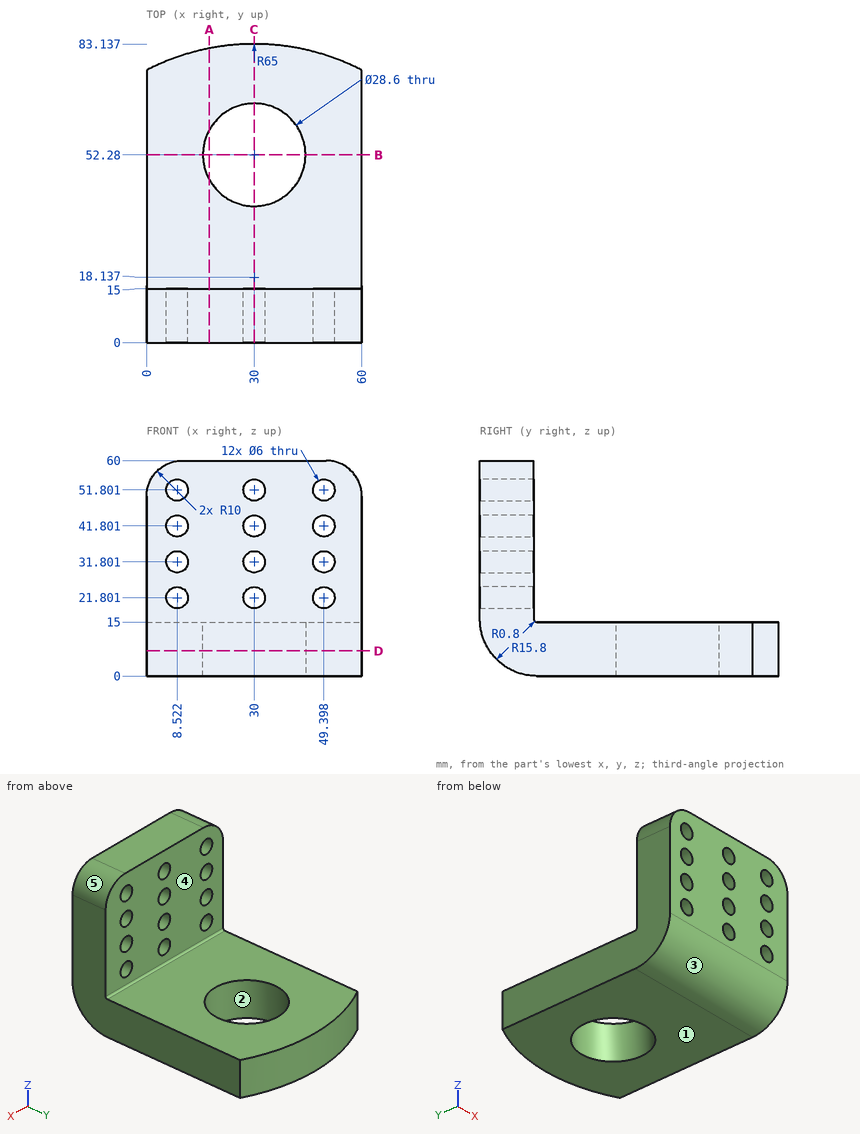
Source: three-view drawing plus pictorial views. Frame: mm from the lowest corner of the part. A direction names the side the tool comes from. Round coordinates to 2 decimals unless told otherwise and drop trailing zeros. Loops run counter-clockwise (first coordinate to the right, second up) from the corner with the lowest first, then second, coordinate; pieces in that order, holes last.
1. Section query B-B on y = 52.28. Output: boundary loops of the cut face in (x, z).
2. Ray query, L1, parallel to X at y = 52, z = 6; L2, parallel to X at y = 8.5, z = 44; L3, parallel to X at y = 11, z = 43. Return the intervals inside material, ascending.
3. Section query A-A on x = 17.5. Output: boundary loops of the cut face in (y, z) (1 decimal), and give its area (3 significant figures).
4. Section query C-C on x = 30. Output: boundary loops of the cut face in (y, z), and give its area (3 significant figures).
5. Mould query, pull axis Y, two halves, no side actions, for the marked faces 1, 2 and 3. Classes: released by +Y, released by -Y, zero draft, split by the parting line, or undercut.
6. Contact query for flat-ended pins moving along their axis: pin 1 (3.5 mm diameter, centred on x = 30, z = 31.8, fed in from -Y) (3 decimals); pin 2 (1.5 mm diameter, centred on x = 38, y = 69, fed in from +Z); pin 3 (7 mm diameter, centred on x = 30, z = 41.8, fed in from +Y); pin 4 (12 mm diameter, centred on x = 18, z = 16.5, fed in from +Y). Output: stop coordinate, or through.
7. Section query D-D on z = 7. Output: boundary loops of the cut face in (x, y), and give its area (3 significant figures).
8. Access query for the marked faces 4 and 5. Directions: +Z, -Z, +X, -X, +Y, -Y. A direction counts if a zero-diameter tool reaches every point of the face in a straight line with its end or side. Return the directions, or none.
Answers below:
1. outline: (0, 0) - (15.7, 0) - (15.7, 15) - (0, 15) - close; (44.3, 0) - (60, 0) - (60, 15) - (44.3, 15) - close
2. L1: x = 0 to 15.7, 44.3 to 60
2. L2: x = 0 to 6.48, 10.56 to 27.96, 32.04 to 47.36, 51.44 to 60
2. L3: x = 0 to 5.77, 11.27 to 27.25, 32.75 to 46.65, 52.15 to 60
3. outline: (0, 15.8) arc R15.8 ccw to (15.8, 0) - (45.3, 0) - (45.3, 15) - (15.8, 15) arc R0.8 cw to (15, 15.8) - (15, 60) - (0, 60) - close; (59.2, 0) - (81.9, 0) - (81.9, 15) - (59.2, 15) - close
3. area: 1,640 mm2
4. outline: (0, 15.8) arc R15.8 ccw to (15.8, 0) - (37.98, 0) - (37.98, 15) - (15.8, 15) arc R0.8 cw to (15, 15.8) - (15, 18.8) - (0, 18.8) - close; (0, 24.8) - (15, 24.8) - (15, 28.8) - (0, 28.8) - close; (0, 34.8) - (15, 34.8) - (15, 38.8) - (0, 38.8) - close; (0, 44.8) - (15, 44.8) - (15, 48.8) - (0, 48.8) - close; (0, 54.8) - (15, 54.8) - (15, 60) - (0, 60) - close; (66.58, 0) - (83.14, 0) - (83.14, 15) - (66.58, 15) - close
4. area: 1,080 mm2
5. face 1: zero draft
5. face 2: undercut
5. face 3: released by -Y
6. pin 1: passes through
6. pin 2: stops at z = 15
6. pin 3: stops at y = 15
6. pin 4: stops at y = 82.84
7. outline: (0, 2.68) - (60, 2.68) - (60, 75.8) arc R65 ccw to (0, 75.8) - close; hole circle Ø28.6 at (30, 52.28)
7. area: 4,040 mm2
8. face 4: +Z, +X, -X, +Y
8. face 5: +Z, +X, +Y, -Y
